For this review, take the finished solid that the model builds, in its own axes (mm). A direction names the side the tool comes from. Round coordinates to 2 decimals unless told otherwise and drop trailing zeros. Loops run counter-clockwise (first coordinate to the right, second up) from the corner with the lowest first, then second, coordinate; pieces in that order, holes last. Notation, with made-up numbers: M 9.25,56 L 25.25,56 A10 ccw 25.25,75 Z; hole C -27.5,77 d11. An arc over 180 degrees is marked long. One line per question, with ' | ' between items. Start each with the question number.
1) Mouldability with a two-part tool opening along Z and no side actions: class faces 4 (the face through (-13.13, 0.84, 6.41)), 5 (the face through (3.755, 19.544, 11.923)), 6 (the face through (0, 0, 0)) as pulls with the +Z half, pulls with the -Z half, needs draft (parallel to the pull), parting line crosses it, or undercut.
2) For faces 1 (the face through (13, 1.7, -9)), 2 (the face through (-24.397, 2.218, 12.69)), 3 (the face through (-12.133, 4.014, 7.89)), list the 3-axis set-ups (+Z, -Z, +X, -X, +Y, -Y) from which the entire face can be reached by the end or side of a thin tool; tool diameter is ignored.
3) For pin 1 Ø6 at (y, z) = (14.5, -1) entering from +X; pin 2 Ø3 at (x, y) = (7.5, 23.5) entering from +Z; pin 3 Ø0.8 at (y, z) = (0.5, -8) entering from +X, all flat-tipped, find the tip position at first contact; note any pin that passes through.
4) We need section A-A (z = -8.15). State how many separate pieces and enclosed holes the cut face has, and give its area (3 significant figures).
5) We need section B-B (y = 11.5). Give the boundary of the cut face in (x, z), and give its area (3 significant figures).
6) For probe 1 along X at (y, z) = (4, -8); probe 2 along X at (y, z) = (2.3, -8.15); probe 3 along Y at (x, z) = (-13, 4), list the stretches that pass through material, from the lowest coordinate up. Write a range as from..to.
```python
from build123d import *

# Parameters (mm, degrees)
SKETCH1_R           = 27.5
BOSS_EXTRUDE1_DEPTH = 5
SKETCH2_R           = 2
CUT_EXTRUDE1_DEPTH  = 2
SKETCH3_R           = 1.25
CUT_EXTRUDE2_DEPTH  = 40.210967853
CUT_EXTRUDE3_DEPTH  = 1.7
SKETCH5_R           = 12.5
BOSS_EXTRUDE2_DEPTH = 30
FILLET1_R           = 0.5


with BuildPart() as part:
    # Sketch1 → Boss-Extrude1 (new body)
    with BuildSketch(Plane(origin=(0, 0, 0), x_dir=(1, 0, 0), z_dir=(0, 1, 0))):
        with Locations(Location((0, 0, 0), (0, 0, 270))):
            Circle(SKETCH1_R)
    extrude(amount=BOSS_EXTRUDE1_DEPTH)

    # Sketch2 → Cut-Extrude1 (cut)
    with BuildSketch(Plane(origin=(0, 5, 0), x_dir=(1, 0, 0), z_dir=(0, 1, 0))):
        with Locations(Location((0, 16.3, 0), (0, 0, 270))):
            Circle(SKETCH2_R)
        with Locations(Location((14.116214082, 8.15, 0), (0, 0, 270))):
            Circle(SKETCH2_R)
        with Locations(Location((14.116214082, -8.15, 0), (0, 0, 270))):
            Circle(SKETCH2_R)
        with Locations(Location((0, -16.3, 0), (0, 0, 270))):
            Circle(SKETCH2_R)
        with Locations(Location((-14.116214082, -8.15, 0), (0, 0, 270))):
            Circle(SKETCH2_R)
        with Locations(Location((-14.116214082, 8.15, 0), (0, 0, 270))):
            Circle(SKETCH2_R)
    extrude(amount=-CUT_EXTRUDE1_DEPTH, mode=Mode.SUBTRACT)

    # Sketch3 → Cut-Extrude2 (cut, through all)
    with BuildSketch(Plane(origin=(0, 5, 0), x_dir=(1, 0, 0), z_dir=(0, 1, 0))):
        with Locations(Location((0, 16.3, 0), (0, 0, 270))):
            Circle(SKETCH3_R)
        with Locations(Location((14.116214082, 8.15, 0), (0, 0, 270))):
            Circle(SKETCH3_R)
        with Locations(Location((14.116214082, -8.15, 0), (0, 0, 270))):
            Circle(SKETCH3_R)
        with Locations(Location((0, -16.3, 0), (0, 0, 270))):
            Circle(SKETCH3_R)
        with Locations(Location((-14.116214082, -8.15, 0), (0, 0, 270))):
            Circle(SKETCH3_R)
        with Locations(Location((-14.116214082, 8.15, 0), (0, 0, 270))):
            Circle(SKETCH3_R)
    extrude(amount=-CUT_EXTRUDE2_DEPTH, mode=Mode.SUBTRACT)

    # Sketch4 → Cut-Extrude3 (cut)
    with BuildSketch(Plane.XZ):
        Polygon((12.116214082, 6.995299462), (14.116214082, 5.840598923), (16.116214082, 6.995299462), (16.116214082, 9.304700538), (14.116214082, 10.459401077), (12.116214082, 9.304700538), align=None)
        Polygon((0, 13.990598923), (2, 15.145299462), (2, 17.454700538), (0, 18.609401077), (-2, 17.454700538), (-2, 15.145299462), align=None)
        Polygon((12.116214082, -6.995299462), (12.116214082, -9.304700538), (14.116214082, -10.459401077), (16.116214082, -9.304700538), (16.116214082, -6.995299462), (14.116214082, -5.840598923), align=None)
        Polygon((0, -13.990598923), (-2, -15.145299462), (-2, -17.454700538), (0, -18.609401077), (2, -17.454700538), (2, -15.145299462), align=None)
        Polygon((-12.116214082, -6.995299462), (-14.116214082, -5.840598923), (-16.116214082, -6.995299462), (-16.116214082, -9.304700538), (-14.116214082, -10.459401077), (-12.116214082, -9.304700538), align=None)
        Polygon((-12.116214082, 6.995299462), (-12.116214082, 9.304700538), (-14.116214082, 10.459401077), (-16.116214082, 9.304700538), (-16.116214082, 6.995299462), (-14.116214082, 5.840598923), align=None)
    extrude(amount=-CUT_EXTRUDE3_DEPTH, mode=Mode.SUBTRACT)

    # Sketch5 → Boss-Extrude2 (add)
    with BuildSketch(Plane(origin=(0, 5, 0), x_dir=(1, 0, 0), z_dir=(0, 1, 0))):
        with Locations(Location((0, 0, 0), (0, 0, 270))):
            Circle(SKETCH5_R)
    extrude(amount=BOSS_EXTRUDE2_DEPTH)

    # Fillet1
    fillet1_edges = [part.edges().sort_by_distance(p)[0] for p in [
        (0, 35, -12.5),
        (0, 5, -27.5),
    ]]
    fillet(fillet1_edges, radius=FILLET1_R)


solid = part.part
```
Answers below:
1) face 4: undercut | face 5: parting line crosses it | face 6: needs draft
2) face 1: -Y | face 2: +Y, -Y | face 3: +Y
3) pin 1: x = 12.5 | pin 2: z = 10.97 | pin 3: x = 26.43
4) separate pieces: 3 | enclosed holes: 0 | area: 795 mm^2
5) outline: C 0,0 d25 | area: 491 mm^2
6) probe 1: -26.31..-16.11, -12.12..12.12, 16.11..26.31 | probe 2: -26.26..-15.37, -12.87..12.87, 15.37..26.26 | probe 3: 0..5
